Input: part model. Units: mm. Frame: model coordinates. Face numbers are marked on the shaded views. A direction names the side the tool comes from. Give positions to 0.01 mm unless a question says otherwise; leave off trailing zeros. Write each loop counter-clockwise with the first axis right and the second up, starting at its lowest first coordinate (ties: lowest second). Pieces come first, ordered by that corner, then holes. Notation, with made-up numbers: (-32, 60.25) - (-8, 60.25) arc R33 cw to (-8, 96.25) - close; hole circle Ø10 at (-31.75, 79). An arc over 180 degrees is marked (long way). Use a Markdown table: item, result. Add a question column.
1. Mould query, pull axis Z, two halves, no side actions, for the marked faces 1, 2 and 3. Classes: released by +Z, released by -Z, zero draft, split by the parting line, or undercut.
2. Section query C-C, the plane x = 0. Return loops of the section in (y, z), plus the area to 3 significant figures.
3. Section query B-B, the plane y = -4.5. Return loops of the section in (x, z), plus the area to 3 significant figures.
4. Section query D-D, the plane z = -12. Return loops of the section in (x, y), plus the area to 3 significant figures.
5. Set-up query: the marked faces 4 and 5. Return all of +Z, -Z, +X, -X, +Y, -Y with unobstructed straight access to the full face (end or side cutting, diameter ignored); none if empty.
6. Section query A-A, the plane z = -112. Return loops of the section in (x, y), plus the area to 3 significant figures.
7. Material intervals for probe 1 along Y at (x, z) = (-3.5, 123); probe 2 along Z at (x, y) = (-8.5, 12); probe 3 along Z at (x, y) = (-12.5, 6), sorted ascending.
8. Pin query (flat end, axial travel): pin 1 (2 mm diameter, centred on x = -22.5, y = -4.5, fed in from +Z); pin 2 (1.5 mm diameter, centred on y = -35.5, z = -80, fed in from -X); pin 3 (24 mm diameter, centred on y = 4.5, z = -18.5, fed in from +X); pin 4 (5 mm diameter, centred on y = -11.5, z = 0, fed in from -X). Return the tip coordinate at first contact, or that it passes through.
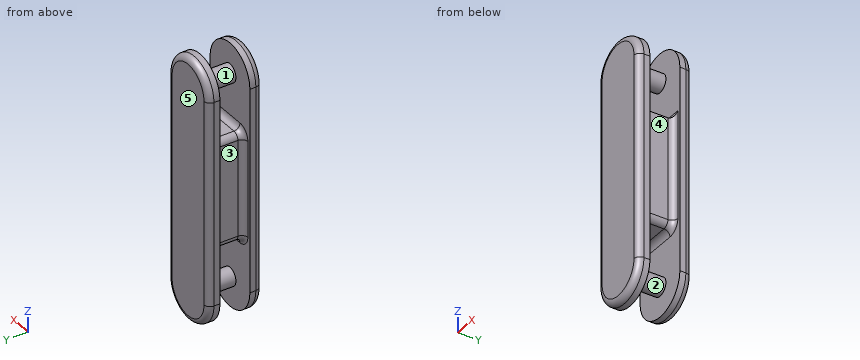
```python
from build123d import *

# Parameters (mm, degrees)
EXTRUDE_1_DEPTH = 20
EXTRUDE_2_DEPTH = 20
SKETCH_3_R      = 15
SKETCH_3_W      = 70
SKETCH_3_H      = 180
EXTRUDE_3_DEPTH = 90
FILLET_1_R      = 10
FILLET_2_R      = 10


with BuildPart() as part:
    # Sketch 1 → Extrude 1 (new body)
    with BuildSketch(Plane(origin=(0, 25, 0), x_dir=(1, 0, 0), z_dir=(0, 1, 0))):
        with BuildLine():
            Line((-50, 170), (-50, -170))
            ThreePointArc((-50, -170), (0, -220), (50, -170))
            Line((50, -170), (50, 170))
            ThreePointArc((50, 170), (0, 220), (-50, 170))
        make_face()
    extrude(amount=EXTRUDE_1_DEPTH)



with BuildPart() as body_2:
    # Sketch 2 → Extrude 2 (new body)
    with BuildSketch(Plane(origin=(0, -25, 0), x_dir=(1, 0, 0), z_dir=(0, 1, 0))):
        with BuildLine():
            Line((50, -170), (50, 170))
            ThreePointArc((50, 170), (0, 220), (-50, 170))
            Line((-50, 170), (-50, -170))
            ThreePointArc((-50, -170), (0, -220), (50, -170))
        make_face()
    extrude(amount=-EXTRUDE_2_DEPTH)


with BuildPart() as part_1:
    add(part.part)

    add(body_2.part)  # Extrude 3 merges body 2
    # Sketch 3 → Extrude 3 (add)
    with BuildSketch(Plane(origin=(0, 45, 0), x_dir=(1, 0, 0), z_dir=(0, 1, 0))):
        with Locations((0, 170)):
            Circle(SKETCH_3_R)
        with Locations((0, -170)):
            Circle(SKETCH_3_R)
        Rectangle(SKETCH_3_W, SKETCH_3_H)
    extrude(amount=-EXTRUDE_3_DEPTH)

    # Fillet 1
    fillet_1_edges = [part_1.edges().sort_by_distance(p)[0] for p in [
        (0, 45, -220),
        (-50, 45, 0),
        (0, -45, -220),
        (50, -45, 0),
        (0, -45, 220),
        (-50, -45, 0),
        (0, 45, 220),
        (50, 45, 0),
    ]]
    fillet(fillet_1_edges, radius=FILLET_1_R)

    # Fillet 2
    fillet_2_edges = [part_1.edges().sort_by_distance(p)[0] for p in [
        (35, -25, 0),
        (35, 0, -90),
        (0, -25, 90),
        (-35, -25, 0),
        (-35, 0, 90),
        (0, -25, -90),
        (-35, 0, -90),
        (35, 25, 0),
        (0, 25, 90),
        (-35, 25, 0),
        (0, 25, -90),
    ]]
    fillet(fillet_2_edges, radius=FILLET_2_R)


solid = part_1.part
```
Result sheet:
| question | item | result |
|---|---|---|
| 1 | face 1 | undercut |
| 1 | face 2 | undercut |
| 1 | face 3 | zero draft |
| 2 | outline | (-45, -210) arc R10 ccw to (-35, -220) - (-25, -220) - (-25, -185) - (25, -185) - (25, -220) - (35, -220) arc R10 ccw to (45, -210) - (45, 210) arc R10 ccw to (35, 220) - (25, 220) - (25, 185) - (-25, 185) - (-25, 220) - (-35, 220) arc R10 ccw to (-45, 210) - close; hole (-25, -155) - (25, -155) - (25, -100) arc R10 ccw to (15, -90) - (-15, -90) arc R10 ccw to (-25, -100) - close; hole (-25, 100) arc R10 ccw to (-15, 90) - (15, 90) arc R10 ccw to (25, 100) - (25, 155) - (-25, 155) - close |
| 2 | area | 29,600 mm² |
| 3 | outline | (-35, -80) arc R10 ccw to (-25, -90) - (25, -90) arc R10 ccw to (35, -80) - (35, 90) - (-25, 90) arc R10 ccw to (-35, 80) - close; circle Ø30 at (0, -170); circle Ø30 at (0, 170) |
| 3 | area | 13,900 mm² |
| 4 | outline | (-50, -35) arc R10 ccw to (-40, -45) - (40, -45) arc R10 ccw to (50, -35) - (50, -25) - (45, -25) arc R10 cw to (35, -15) - (35, 15) arc R10 cw to (45, 25) - (50, 25) - (50, 35) arc R10 ccw to (40, 45) - (-40, 45) arc R10 ccw to (-50, 35) - (-50, 25) - (-45, 25) arc R10 cw to (-35, 15) - (-35, -15) arc R10 cw to (-45, -25) - (-50, -25) - close |
| 4 | area | 7,500 mm² |
| 5 | face 4 | +Z, -Z, +X |
| 5 | face 5 | +Z, -Z, +X, -X, +Y |
| 6 | outline | (-50, -35) arc R10 ccw to (-40, -45) - (40, -45) arc R10 ccw to (50, -35) - (50, -25) - (-50, -25) - close; (-50, 25) - (50, 25) - (50, 35) arc R10 ccw to (40, 45) - (-40, 45) arc R10 ccw to (-50, 35) - close |
| 6 | area | 3,910 mm² |
| 7 | probe 1 | y = -45 to -25, 25 to 45 |
| 7 | probe 2 | z = -182.36 to -157.64, -90 to 90, 157.64 to 182.36 |
| 7 | probe 3 | z = -178.29 to -161.71, -90 to 90, 161.71 to 178.29 |
| 8 | pin 1 | stops at z = 90 |
| 8 | pin 2 | stops at x = -50 |
| 8 | pin 3 | stops at x = 35.11 |
| 8 | pin 4 | stops at x = -35 |
